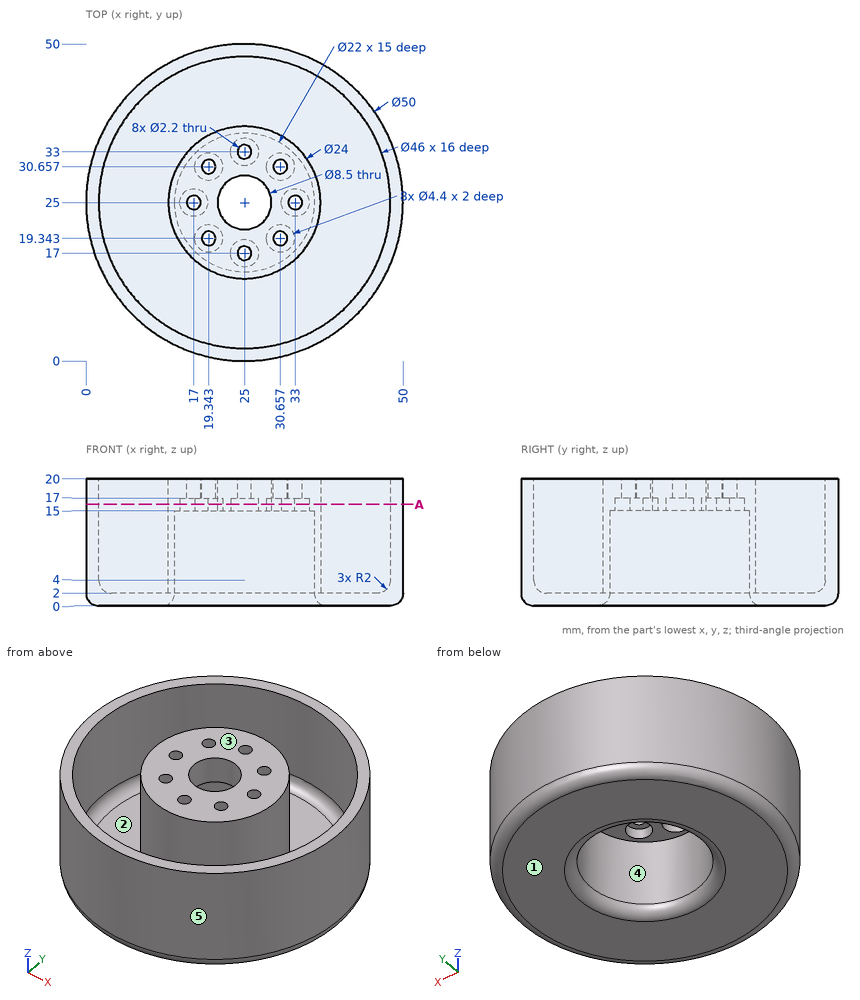
Could you check a few things on this drawing? It's one solid part, dimensions in mm from its lowest x, y, z. A direction names the side the tool comes from. Coordinates: 2 decimals unless noted, no trailing zeros.
1. I'm going to push flat-ended pins straight in: pin 1 (1 mm diameter, centred on y = 31, z = 9.5, fed in from +X); pin 2 (12 mm diameter, centred on x = 20, y = 20.5, fed in from -Z); pin 3 (1 mm diameter, centred on x = 9.5, z = 7, fed in from +Y). Where does each tip first touch, or does it pass through?
2. For the marked faces 1 and 2, which set-ups out of +Z, -Z, +X, -X, +Y, -Y let a thin tool reach every point of the face, with its end or its side?
3. I need wall thicknesses on line 1 (Y direction, x = 25, z = 14.5); line 2 (Y direction, x = 23, z = 11); line 3 (X direction, y = 31.5, z = 6). Which ranges of each line are inside material? Lowest first, please.
4. If we section it at A-A (z = 16): Give the number of separate pieces and of enclosed holes in the cut face.
5. Thinking about a two-plate mould opening in Y: for the marked faces 3, 4 and 5, which applies, +Y half, -Y half, draft (parallel to the pull), parting line (faces both ways), or undercut?
Entries:
1. pin 1: stops at x = 49.39
1. pin 2: stops at z = 0.02
1. pin 3: stops at y = 45
2. face 1: -Z, +X, -X, +Y, -Y
2. face 2: +Z
3. line 1: y = 0 to 2, 13 to 14, 36 to 37, 48 to 50
3. line 2: y = 0.08 to 2.09, 13.17 to 14.18, 35.82 to 36.83, 47.91 to 49.92
3. line 3: x = 0.86 to 2.94, 14.91 to 16.13, 33.87 to 35.09, 47.06 to 49.14
4. separate pieces: 2
4. enclosed holes: 10
5. face 3: draft
5. face 4: undercut
5. face 5: parting line
